```python
from build123d import *

# Parameters (mm, degrees)
SKETCH_1_W           = 54.61
SKETCH_1_H           = 29.97
EXTRUDE_1_DEPTH      = 2.5
EXTRUDE_2_DEPTH      = 17
CUT_EXTRUDE_1_DEPTH  = 30.97
SKETCH_4_R           = 1.145
CUT_EXTRUDE_2_DEPTH  = 3.5
SKETCH_5_R           = 2.25
SKETCH_5_W           = 7.5
SKETCH_5_H           = 6
SKETCH_5_W_2         = 9.5
EXTRUDE_3_DEPTH      = 1.12
SKETCH_6_R           = 1.145
CUT_EXTRUDE_3_DEPTH  = 4.62
SKETCH_7_R           = 1.5
CUT_EXTRUDE_4_DEPTH  = 1
EXTRUDE_4_DEPTH      = 9.5
EXTRUDE_4_DEPTH_BACK = 9.5
SKETCH_9_W           = 0.66
SKETCH_9_H           = 0.76
EXTRUDE_5_DEPTH      = 3
SKETCH_10_R          = 3.75
EXTRUDE_6_DEPTH      = 1
SKETCH_11_R          = 3
SKETCH_11_R_2        = 2
EXTRUDE_7_DEPTH      = 4
SKETCH_12_R          = 4.25
SKETCH_12_R_2        = 3.25
EXTRUDE_8_DEPTH      = 4


with BuildPart() as part:
    # Эскиз1 → Бобышка-Вытянуть1 (new body)
    with BuildSketch(Plane(origin=(0, 0, 0), x_dir=(1, 0, 0), z_dir=(0, 1, 0))):
        Rectangle(SKETCH_1_W, SKETCH_1_H)
    extrude(amount=EXTRUDE_1_DEPTH)

    # Эскиз2 → Бобышка-Вытянуть2 (add)
    with BuildSketch(Plane(origin=(0, 2.5, 0), x_dir=(1, 0, 0), z_dir=(0, 1, 0))):
        with BuildLine():
            Line((27.305, -14.985), (-0.695, -14.985))
            Line((-0.695, -14.985), (-0.695, -13.485))
            Line((-0.695, -13.485), (23.305, -13.485))
            ThreePointArc((23.305, -13.485), (24.719213562, -12.899213562), (25.305, -11.485))
            Line((25.305, -11.485), (25.305, 11.485))
            ThreePointArc((25.305, 11.485), (24.719213562, 12.899213562), (23.305, 13.485))
            Line((23.305, 13.485), (-0.695, 13.485))
            Line((-0.695, 13.485), (-0.695, 14.985))
            Line((-0.695, 14.985), (27.305, 14.985))
            Line((27.305, 14.985), (27.305, -14.985))
        make_face()
    extrude(amount=EXTRUDE_2_DEPTH)

    # Эскиз3 → Вырез-Вытянуть1 (cut, through all)
    with BuildSketch(Plane.XY.offset(14.985)):
        Polygon((-0.695, 2.5), (25.305, 19.5), (-0.695, 19.5), align=None)
    extrude(amount=-CUT_EXTRUDE_1_DEPTH, mode=Mode.SUBTRACT)

    # Эскиз4 → Вырез-Вытянуть2 (cut, through all)
    with BuildSketch(Plane(origin=(0, 2.5, 0), x_dir=(1, 0, 0), z_dir=(0, 1, 0))):
        with Locations((-13.495, 11.175)):
            Circle(SKETCH_4_R)
        with Locations((-0.005, -11.175)):
            Circle(SKETCH_4_R)
        with Locations((13.475, 11.175)):
            Circle(SKETCH_4_R)
    extrude(amount=-CUT_EXTRUDE_2_DEPTH, mode=Mode.SUBTRACT)

    # Эскиз5 → Бобышка-Вытянуть3 (add)
    with BuildSketch(Plane.XZ):
        with Locations((-0.005, 11.175)):
            Circle(SKETCH_5_R)
        with Locations((13.475, -11.175)):
            Circle(SKETCH_5_R)
        with Locations((-13.495, -11.175)):
            Circle(SKETCH_5_R)
        with Locations((-23.555, 11.985)):
            Rectangle(SKETCH_5_W, SKETCH_5_H)
        with Locations((22.555, 11.985)):
            Rectangle(SKETCH_5_W_2, SKETCH_5_H)
        with Locations((22.555, -11.985)):
            Rectangle(SKETCH_5_W_2, SKETCH_5_H)
        with Locations((-23.555, -11.985)):
            Rectangle(SKETCH_5_W, SKETCH_5_H)
    extrude(amount=EXTRUDE_3_DEPTH)

    # Эскиз6 → Вырез-Вытянуть3 (cut, through all)
    with BuildSketch(Plane(origin=(0, 2.5, 0), x_dir=(1, 0, 0), z_dir=(0, 1, 0))):
        with Locations((-13.495, 11.175)):
            Circle(SKETCH_6_R)
        with Locations((13.475, 11.175)):
            Circle(SKETCH_6_R)
        with Locations((-0.005, -11.175)):
            Circle(SKETCH_6_R)
    extrude(amount=-CUT_EXTRUDE_3_DEPTH, mode=Mode.SUBTRACT)

    # Эскиз7 → Вырез-Вытянуть4 (cut)
    with BuildSketch(Plane(origin=(0, 2.5, 0), x_dir=(1, 0, 0), z_dir=(0, 1, 0))):
        with Locations((-13.495, 11.175)):
            Circle(SKETCH_7_R)
        with Locations((13.475, 11.175)):
            Circle(SKETCH_7_R)
        with Locations((-0.005, -11.175)):
            Circle(SKETCH_7_R)
    extrude(amount=-CUT_EXTRUDE_4_DEPTH, mode=Mode.SUBTRACT)

    # Эскиз8 → Бобышка-Вытянуть4 (add, two sides)
    with BuildSketch(Plane.XY) as extrude_4_sk:
        Polygon((-27.305, 2.5), (-24.695, 13.85), (-23.695, 11.232050808), (-24.695, 9.5), (-24.695, 2.5), align=None)
    extrude(amount=EXTRUDE_4_DEPTH)
    extrude(extrude_4_sk.sketch, amount=-EXTRUDE_4_DEPTH_BACK)

    # Эскиз9 → Бобышка-Вытянуть5 (add)
    with BuildSketch(Plane.XZ):
        with Locations((25.075, 6.35)):
            Rectangle(SKETCH_9_W, SKETCH_9_H)
        with Locations((25.075, -6.35)):
            Rectangle(SKETCH_9_W, SKETCH_9_H)
    extrude(amount=EXTRUDE_5_DEPTH)

    # Эскиз10 → Бобышка-Вытянуть6 (add)
    with BuildSketch(Plane.ZY.offset(-25.305)):
        with Locations((-6.35, 11.48)):
            Circle(SKETCH_10_R)
        with Locations((6.35, 11.48)):
            Circle(SKETCH_10_R)
    extrude(amount=EXTRUDE_6_DEPTH)

    # Эскиз11 → Бобышка-Вытянуть7 (add)
    with BuildSketch(Plane.ZY.offset(-24.305)):
        with Locations((-6.35, 11.48)):
            Circle(SKETCH_11_R)
        with Locations((-6.35, 11.48)):
            Circle(SKETCH_11_R_2, mode=Mode.SUBTRACT)
    extrude(amount=EXTRUDE_7_DEPTH)

    # Эскиз12 → Бобышка-Вытянуть8 (add)
    with BuildSketch(Plane.ZY.offset(-24.305)):
        with Locations((6.35, 11.48)):
            Circle(SKETCH_12_R)
        with Locations((6.35, 11.48)):
            Circle(SKETCH_12_R_2, mode=Mode.SUBTRACT)
    extrude(amount=EXTRUDE_8_DEPTH)


solid = part.part
```
Check sheet for the modelled part. Datum: model origin and axes. Units: mm. A direction names the side the tool comes from. Round coordinates to 2 decimals unless told otherwise and drop trailing zeros. Order: outer loops, then holes, each group sorted by start corner. A loop starts at its lowest first (then second) coordinate and runs counter-clockwise, first axis right, second up. Notation, with made-up numbers: M 33,72 L 41,72 A30 ccw 41,97 Z; hole C -31,-31 d3. An arc over 180 degrees is marked long. Answer in a Markdown table with one row per item.
(1) Material ranges on line 1 along Z through (x, y) = (13.5, 5) (3 decimals); line 2 along Z through (x, y) = (-21.5, -0.5) (3 decimals); line 3 along Y through (x, z) = (23, 8), recorded low to high. Write a range as from..to.
Findings:
| item | result |
|---|---|
| line 1 | z = -14.985..-13.485, 13.485..14.985 |
| line 2 | z = -14.985..-8.985, 8.985..14.985 |
| line 3 | y = 0..2.5, 7.56..8.68, 14.28..15.4 |
(2) Set-up check for faces 1 (the cylindrical face through (24.704, 10.881, 12.915)), 2 (the flat face through (24.305, 12, -6)), 3 (the cylindrical face through (12.285, 2.007, -10.262)), 4 (the flat face through (22.5, -0.6, -8.985)): record each of +Z, -Z, +X, -X, +Y, -Y from which the full face is reachable in a straight line by a thin tool's end or side.
Findings:
| item | result |
|---|---|
| face 1 | -X, +Y |
| face 2 | none |
| face 3 | +Y |
| face 4 | +X, -Y |
(3) Section check A-A on y = 17. Record the boundary of the cut face in (x, z) (3 decimals), plus the area to 3 significant figures.
Findings:
| item | result |
|---|---|
| outline | M 21.481,-14.985 L 27.305,-14.985 L 27.305,14.985 L 21.481,14.985 L 21.481,13.485 L 23.305,13.485 A2 cw 25.305,11.485 L 25.305,-11.485 A2 cw 23.305,-13.485 L 21.481,-13.485 Z |
| area | 73.1 mm^2 |
(4) Section check C-C on x = 3. Record the boundary of the cut face in (y, z) (3 decimals), plus the area to 3 significant figures.
Findings:
| item | result |
|---|---|
| outline | M 0,-14.985 L 4.916,-14.985 L 4.916,-13.485 L 2.5,-13.485 L 2.5,13.485 L 4.916,13.485 L 4.916,14.985 L 0,14.985 Z |
| area | 82.2 mm^2 |
(5) Draft check along Z on faces 5 (the cylindrical face through (22.333, 12.832, -7.824)), 6 (the flat face through (17.805, -0.6, 11.9)), 7 (the cylindrical face through (-0.253, 0.208, 12.293)), 8 (the flat face through (-25, 7, -9.5)). Enter one of: +Z half, -Z half, draft (parallel to the pull), parting line (faces both ways), or undercut.
Findings:
| item | result |
|---|---|
| face 5 | undercut |
| face 6 | draft |
| face 7 | undercut |
| face 8 | -Z half |
(6) Section check B-B on x = 18.5. Record the boundary of the cut face in (y, z) (3 decimals).
Findings:
| item | result |
|---|---|
| outline | M -1.12,-14.985 L 15.051,-14.985 L 15.051,-13.485 L 2.5,-13.485 L 2.5,13.485 L 15.051,13.485 L 15.051,14.985 L -1.12,14.985 L -1.12,8.985 L 0,8.985 L 0,-8.985 L -1.12,-8.985 Z |
(7) Gauge pin test, flat ends, axial feed: pin 1 (3 mm diameter, centred on x = -26, y = 9.5, fed in from +Z); pin 2 (5 mm diameter, centred on x = 0.5, z = 12, fed in from -Y); pin 3 (1 mm diameter, centred on x = -5.5, z = 5.5, fed in from -Y). Record the tip position at first contact, or that the pin passes through.
Findings:
| item | result |
|---|---|
| pin 1 | stops at z = 9.5 |
| pin 2 | stops at y = -1.12 |
| pin 3 | stops at y = 0 |
